For this review, use the dimensioned drawing (mm, ordinates from the lowest corner) and the shaded views. A direction names the side the tool comes from. Coordinates: 2 decimals unless noted, no trailing zeros. Loops run counter-clockwise (first coordinate to the right, second up) from the corner with the lowest first, then second, coordinate; pieces in that order, holes last. Notation, with made-up numbers: M 59.25,43.25 L 98.25,43.25 A4 cw 98.25,50.25 Z; hole C 32,36 d10. An arc over 180 degrees is marked long. Write item = value, one per line. Start each with the question number.
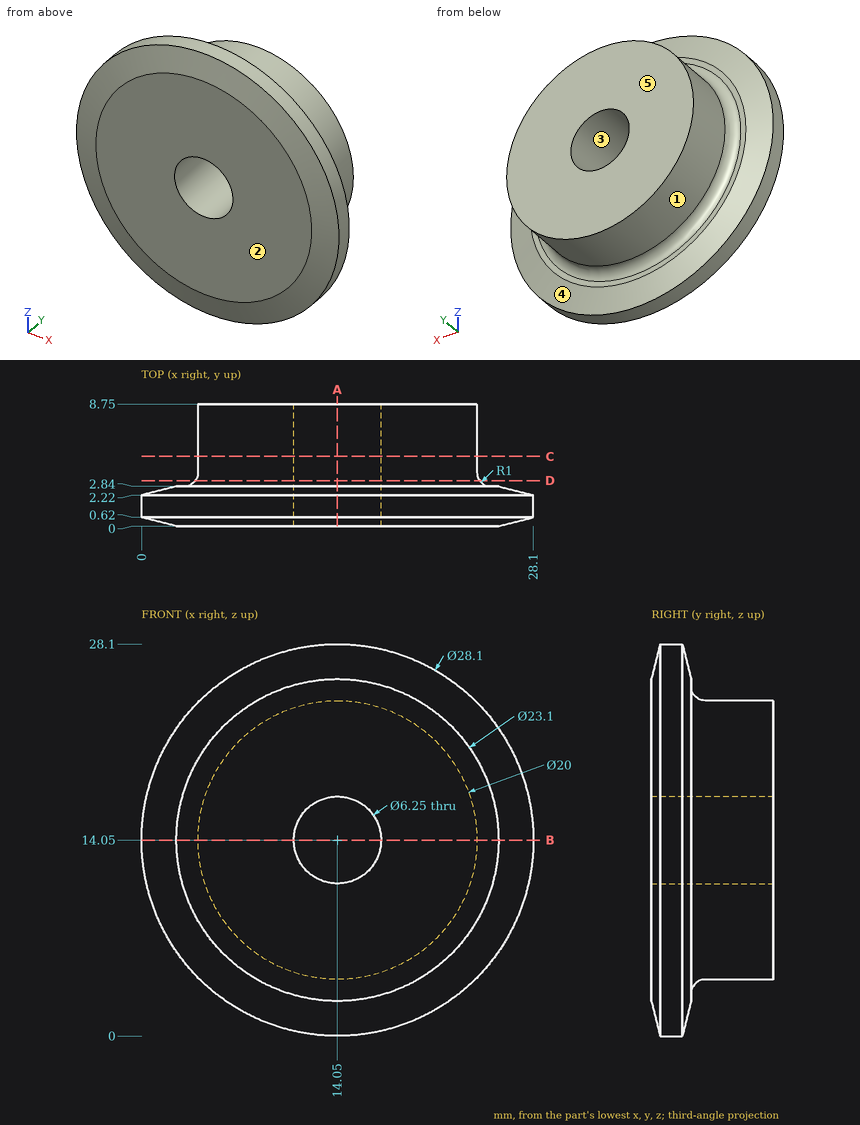
Q1. To check wall thickness, follow line 1 (X direction, y = 4, z = 14.05) (3 decimals); line 2 (Y direction, x = 18, z = 24.75); line 3 (X direction, y = 3, z = 14.05) (3 decimals). State the ranges of each line that lie inside material, in increasing order. Write a range as from..to.
Q2. For the marked faces 1 and 2, list the 3-axis set-ups (+Z, -Z, +X, -X, +Y, -Y) from which the entire face can be reached by the end or side of a thin tool; tool diameter is ignored.
Q3. Add section B-B on z = 14.05. State the section outline as (x, y) points (3 decimals), plus the area to 3 significant figures.
Q4. Add section D-D on y = 3.25. State the section outline as (x, z) points (3 decimals).
Q5. Mouldability with a two-part tool opening along Z and no side actions: class the marked faces 3, 4 and 5 as released by +Z, released by -Z, zero draft, split by the parting line, or undercut.
Q6. Add section C-C on y = 5. State the section outline as (x, z) points (3 decimals), plus the area to 3 significant figures.
Q7. Clearance check with flat-ended pins moving along their axes: P1, Ø4, axis at x = 6.5, z = 22, coming from the +Y side; P2, Ø1, axis at y = 3.5, z = 20.5, coming from the -X side; P3, Ø3, axis at x = 7.5, y = 2.5, coming from the -Z side; P4, Ø5, axis at x = 9.5, y = 5.5, coming from the -Z side. State where each tip first meets the part, or that it passes through.
Q8. Add section A-A on x = 14.05. State the section outline as (y, z) points (3 decimals), plus the area to 3 significant figures.
Values follow:
q1.line_1 = 4.05..10.925, 17.175..24.05
q1.line_2 = 0..2.84
q1.line_3 = 3.593..10.925, 17.175..24.507
q2.face_1 = +Y
q2.face_2 = +Z, -Z, +X, -X, -Y
q3.outline = M 0,0.62 L 2.5,0 L 10.925,0 L 10.925,8.75 L 4.05,8.75 L 4.05,3.84 A1 cw 3.05,2.84 L 2.5,2.84 L 0,2.22 Z; M 17.175,0 L 25.6,0 L 28.1,0.62 L 28.1,2.22 L 25.6,2.84 L 25.05,2.84 A1 cw 24.05,3.84 L 24.05,8.75 L 17.175,8.75 Z
q3.area = 141 mm2
q4.outline = C 14.05,14.05 d20.385; hole C 14.05,14.05 d6.25
q5.face_3 = undercut
q5.face_4 = split by the parting line
q5.face_5 = zero draft
q6.outline = C 14.05,14.05 d20; hole C 14.05,14.05 d6.25
q6.area = 283 mm2
q7.P1 = 8.75
q7.P2 = 5.74
q7.P3 = 0.95
q7.P4 = 4.26
q8.outline = M 0,2.5 L 0.62,0 L 2.22,0 L 2.84,2.5 L 2.84,3.05 A1 cw 3.84,4.05 L 8.75,4.05 L 8.75,10.925 L 0,10.925 Z; M 0,17.175 L 8.75,17.175 L 8.75,24.05 L 3.84,24.05 A1 cw 2.84,25.05 L 2.84,25.6 L 2.22,28.1 L 0.62,28.1 L 0,25.6 Z
q8.area = 141 mm2
